The drawing under review shows one solid part. Ordinate dimensions are in mm from its lowest x, y, z. A direction names the side the tool comes from. Give positions to 0.01 mm unless a question says otherwise; leave off trailing zeros. Loops run counter-clockwise (first coordinate to the right, second up) from the corner with the lowest first, then second, coordinate; pieces in that order, holes last. Notation, with made-up numbers: (37.5, 56) - (82.5, 56) arc R30 cw to (82.5, 91) - close; hole circle Ø1 at (75, 22). An arc over 180 degrees is marked (long way). Return JSON: item names as keys, results as strings. Group by question number.
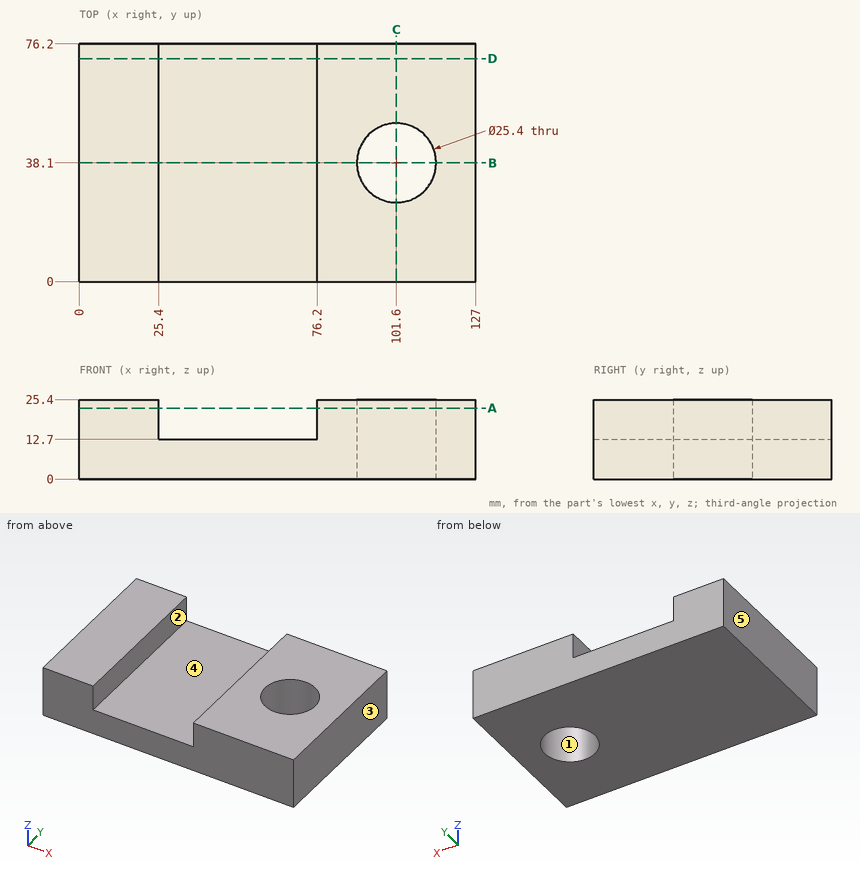
1) We need section B-B, the plane y = 38.1. Write out the cut boundary in (x, z), plus the area to 3 significant figures.
2) We need section A-A, the plane z = 22.75. Write out the cut boundary in (x, y).
3) To check wall thickness, follow line 1 (X direction, y = 37.5, z = 13.75); line 2 (X direction, y = 8, z = 21); line 3 (Y direction, x = 101.6, z = 15.75). State the ranges of each line that lie inside material, in increasing order.
4) We need section D-D, the plane y = 71.5. Write out the cut boundary in (x, z), plus the area to 3 significant figures.
5) Tool access review of the marked faces 1 and 2: name each direction out of +Z, -Z, +X, -X, +Y, -Y from which nothing blocks a thin tool from reaching the whole face with its end or side.
6) Draft analysis for pull direction X (two halves, no side actions). For the marked faces 3, 4 and 5, state which applies: +X half, -X half, draft (parallel to the pull), parting line (faces both ways), or undercut.
7) We need section C-C, the plane x = 101.6. Write out the cut boundary in (y, z).
8) For pin 1 Ø15 at (x, y) = (42, 45) entering from +Z, flat-tipped, find the tip position at first contact; note if it passes through.
Findings:
{
 "1": {"outline": "(0, 0) - (88.9, 0) - (88.9, 25.4) - (76.2, 25.4) - (76.2, 12.7) - (25.4, 12.7) - (25.4, 25.4) - (0, 25.4) - close; (114.3, 0) - (127, 0) - (127, 25.4) - (114.3, 25.4) - close", "area": "1,940 mm^2"},
 "2": {"outline": "(0, 0) - (25.4, 0) - (25.4, 76.2) - (0, 76.2) - close; (76.2, 0) - (127, 0) - (127, 76.2) - (76.2, 76.2) - close; hole circle Ø25.4 at (101.6, 38.1)"},
 "3": {"line 1": "x = 0 to 25.4, 76.2 to 88.91, 114.29 to 127", "line 2": "x = 0 to 25.4, 76.2 to 127", "line 3": "y = 0 to 25.4, 50.8 to 76.2"},
 "4": {"outline": "(0, 0) - (127, 0) - (127, 25.4) - (76.2, 25.4) - (76.2, 12.7) - (25.4, 12.7) - (25.4, 25.4) - (0, 25.4) - close", "area": "2,580 mm^2"},
 "5": {"face 1": "+Z, -Z", "face 2": "+Z, +Y, -Y"},
 "6": {"face 3": "+X half", "face 4": "undercut", "face 5": "-X half"},
 "7": {"outline": "(0, 0) - (25.4, 0) - (25.4, 25.4) - (0, 25.4) - close; (50.8, 0) - (76.2, 0) - (76.2, 25.4) - (50.8, 25.4) - close"},
 "8": {"pin 1": "stops at z = 12.7"}
}
